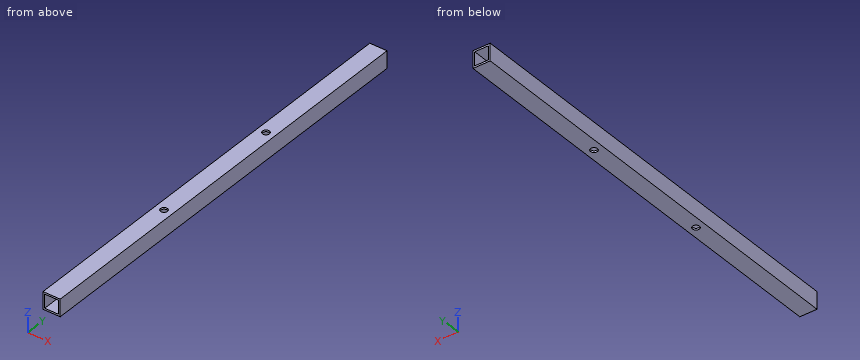
```python
from build123d import *

# Parameters (mm, degrees)
SKETCH_1_W            = 10
SKETCH_1_H            = 10
SKETCH_1_W_2          = 8
SKETCH_1_H_2          = 8
EXTRUDE_1_DEPTH       = 250
HOLE_WIZARD_4_0_4_1_D = 4


with BuildPart() as part:
    # 草图1 → 凸台-拉伸1 (new body)
    with BuildSketch(Plane(origin=(0, 0, 0), x_dir=(1, 0, 0), z_dir=(0, 1, 0))):
        Rectangle(SKETCH_1_W, SKETCH_1_H)
        Rectangle(SKETCH_1_W_2, SKETCH_1_H_2, mode=Mode.SUBTRACT)
    extrude(amount=EXTRUDE_1_DEPTH)

    # Ø4.0 (4) 直径孔1 (through all)
    with Locations(Plane(origin=(0, 0, -5), x_dir=(-1, 0, 0), z_dir=(0, 0, -1))):
        with Locations((0, 164)):
            hole_wizard_4_0_4_1 = Hole(HOLE_WIZARD_4_0_4_1_D / 2)

    # 镜向1: Ø4.0 (4) 直径孔1 across plane
    add(hole_wizard_4_0_4_1.mirror(Plane.ZX.offset(125)), mode=Mode.SUBTRACT)


solid = part.part
```
CAD build for the part. Positions are in the model's coordinates, mm. Coordinates: 2 decimals unless noted, no trailing zeros. Write each loop counter-clockwise with the first axis right and the second up, starting at its lowest first coordinate (ties: lowest second). Pieces come first, ordered by that corner, then holes.
(1) Cut at A-A, the plane y = 148. List the corners of the cut face in (x, z), and give its area (3 significant figures).
(2) Drill centre lines: probe 1 along Y at (x, z) = (0, 4.5); probe 2 along Z at (x, y) = (3.75, 198). Where is each one in solid material? Low to high.
(3) Cut at B-B, the plane x = 0. List the corners of the cut face in (y, z), and give its area (3 significant figures).
(4) Cut at C-C, the plane z = -0.25. List the corners of the cut face in (x, y).
Geometry says:
1. outline: (-5, -5) - (5, -5) - (5, 5) - (-5, 5) - close; hole (-4, -4) - (4, -4) - (4, 4) - (-4, 4) - close
1. area: 36.0 mm2
2. probe 1: y = 0 to 84, 88 to 162, 166 to 250
2. probe 2: z = -5 to -4, 4 to 5
3. outline: (0, -5) - (84, -5) - (84, -4) - (0, -4) - close; (0, 4) - (84, 4) - (84, 5) - (0, 5) - close; (88, -5) - (162, -5) - (162, -4) - (88, -4) - close; (88, 4) - (162, 4) - (162, 5) - (88, 5) - close; (166, -5) - (250, -5) - (250, -4) - (166, -4) - close; (166, 4) - (250, 4) - (250, 5) - (166, 5) - close
3. area: 484 mm2
4. outline: (-5, 0) - (-4, 0) - (-4, 250) - (-5, 250) - close; (4, 0) - (5, 0) - (5, 250) - (4, 250) - close
